from build123d import *

# Parameters (mm, degrees)
DODANIE_WYCI_GNI_CIE1_DEPTH   = 10
SZKIC1_W                      = 5
SZKIC1_H                      = 6
DODANIE_WYCI_GNI_CIE1_2_DEPTH = 10
DODANIE_WYCI_GNI_CIE1_3_DEPTH = 10
SZKIC1_3_W                    = 5
SZKIC1_3_H                    = 5
DODANIE_WYCI_GNI_CIE2_DEPTH   = 5
SZKIC2_R                      = 1
WYTNIJ_WYCI_GNI_CIE1_DEPTH    = 104.949507791


with BuildPart() as part:
    # Szkic1 → Dodanie-wyci_gni_cie1 (new body)
    with BuildSketch(Plane(origin=(0, 0, 0), x_dir=(1, 0, 0), z_dir=(0, 1, 0))):
        with BuildLine():
            Line((-9.449286184, 87.638462845), (9.449286184, 87.638462845))
            ThreePointArc((9.449286184, 87.638462845), (10.74338141, 87.468091977), (11.949286184, 86.968589864))
            Line((11.949286184, 86.968589864), (47.5, 66.443375673))
            ThreePointArc((47.5, 66.443375673), (49.330127019, 64.613248654), (50, 62.113248654))
            Line((50, 62.113248654), (50, 11))
            Line((50, 11), (55, 11))
            Line((55, 11), (55, 89.638462845))
            ThreePointArc((55, 89.638462845), (53.535533906, 93.173996751), (50, 94.638462845))
            Line((50, 94.638462845), (-50, 94.638462845))
            ThreePointArc((-50, 94.638462845), (-53.535533906, 93.173996751), (-55, 89.638462845))
            Line((-55, 89.638462845), (-55, 11))
            Line((-55, 11), (-50, 11))
            Line((-50, 11), (-50, 62.113248654))
            ThreePointArc((-50, 62.113248654), (-49.330127019, 64.613248654), (-47.5, 66.443375673))
            Line((-47.5, 66.443375673), (-11.949286184, 86.968589864))
            ThreePointArc((-11.949286184, 86.968589864), (-10.74338141, 87.468091977), (-9.449286184, 87.638462845))
        make_face()
        with BuildLine():
            ThreePointArc((-48.5, 70.620674679), (-49.5, 70.620674679), (-50, 71.486700083))
            Line((-50, 71.486700083), (-50, 86.638462845))
            ThreePointArc((-50, 86.638462845), (-49.707106781, 87.345569627), (-49, 87.638462845))
            Line((-49, 87.638462845), (-22.756377072, 87.638462845))
            ThreePointArc((-22.756377072, 87.638462845), (-21.790451246, 86.89728189), (-22.256377072, 85.772437442))
            Line((-22.256377072, 85.772437442), (-48.5, 70.620674679))
        make_face(mode=Mode.SUBTRACT)
        with BuildLine():
            Line((48.5, 70.620674679), (22.256377072, 85.772437442))
            ThreePointArc((22.256377072, 85.772437442), (21.790451246, 86.89728189), (22.756377072, 87.638462845))
            Line((22.756377072, 87.638462845), (49, 87.638462845))
            ThreePointArc((49, 87.638462845), (49.707106781, 87.345569627), (50, 86.638462845))
            Line((50, 86.638462845), (50, 71.486700083))
            ThreePointArc((50, 71.486700083), (49.5, 70.620674679), (48.5, 70.620674679))
        make_face(mode=Mode.SUBTRACT)
    extrude(amount=DODANIE_WYCI_GNI_CIE1_DEPTH)



with BuildPart() as body_2:
    # Szkic1 → Dodanie-wyci_gni_cie1 2 (new body)
    with BuildSketch(Plane(origin=(0, 0, 0), x_dir=(1, 0, 0), z_dir=(0, 1, 0))):
        with Locations((52.5, 3)):
            Rectangle(SZKIC1_W, SZKIC1_H)
    extrude(amount=DODANIE_WYCI_GNI_CIE1_2_DEPTH)


with BuildPart() as body_3:
    # Szkic1 → Dodanie-wyci_gni_cie1 3 (new body)
    with BuildSketch(Plane(origin=(0, 0, 0), x_dir=(1, 0, 0), z_dir=(0, 1, 0))):
        with Locations((-52.5, 3)):
            Rectangle(SZKIC1_W, SZKIC1_H)
    extrude(amount=DODANIE_WYCI_GNI_CIE1_3_DEPTH)


with BuildPart() as part_1:
    add(part.part)

    add(body_2.part)  # Dodanie-wyci_gni_cie2 merges body 2

    add(body_3.part)  # Dodanie-wyci_gni_cie2 merges body 3
    # Szkic1_3 → Dodanie-wyci_gni_cie2 (add)
    with BuildSketch(Plane(origin=(0, 0, 0), x_dir=(1, 0, 0), z_dir=(0, 1, 0))):
        with Locations((-52.5, 8.5)):
            Rectangle(SZKIC1_3_W, SZKIC1_3_H)
        with Locations((52.5, 8.5)):
            Rectangle(SZKIC1_3_W, SZKIC1_3_H)
    extrude(amount=DODANIE_WYCI_GNI_CIE2_DEPTH)

    # Szkic2 → Wytnij-wyci_gni_cie1 (cut, through all)
    with BuildSketch(Plane.XY.offset(-87.638462845)):
        with Locations((0, 5)):
            Circle(SZKIC2_R)
    extrude(amount=-WYTNIJ_WYCI_GNI_CIE1_DEPTH, mode=Mode.SUBTRACT)


solid = part_1.part
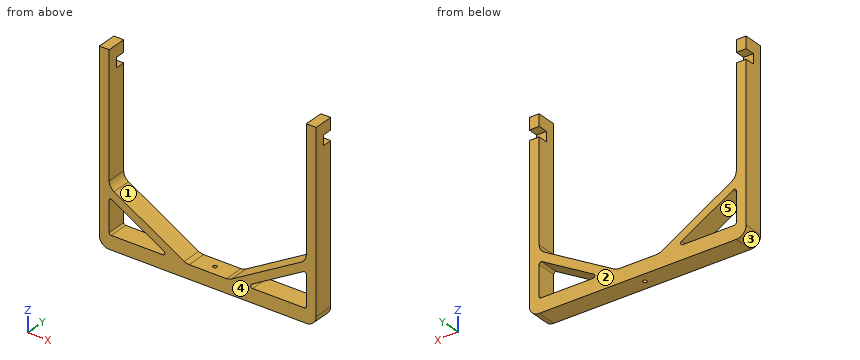
Work out the finished part from the listing and answer in its coordinate system (mm). Face numbers are marked on the shaded views. A direction names the side the tool comes from. Round coordinates to 2 decimals unless told otherwise and drop trailing zeros. Write each loop counter-clockwise with the first axis right and the second up, starting at its lowest first coordinate (ties: lowest second). Pieces come first, ordered by that corner, then holes. Notation, with made-up numbers: (21, 86.5) -> (69, 86.5) arc R19 cw to (69, 90.5) -> close; hole circle Ø11 at (-13, -26). An arc over 180 degrees is marked (long way). Answer as CSV lines item,"result". Start each with the question number.
(1) Each of these flat-tipped pins is pushed along its axis until it touches: pin 1 (1.5 mm diameter, centred on x = 52.5, y = 7, fed in from -Z); pin 2 (6 mm diameter, centred on x = -29.5, y = 4.5, fed in from +Z); pin 3 (5 mm diameter, centred on x = -1, y = 3.5, fed in from +Z). Where does it stop, or does it pass through?
(2) The part is cut by section C-C, the plane x = 4.5. Give the vertices of the cut face in (y, z), then the cut area to 3 significant figures.
(3) A tool of negligible diameter and unlimited length cuts with its end or side. For the marked faces 1 and 2, from which of +Z, -Z, +X, -X, +Y, -Y can it reach the whole face along a straight path? Write none if from no direction.
(4) The part is cut by section A-A, the plane z = -32. Give the vertices of the cut face in (x, y).
(5) The part is cut by section B-B, the plane z = -79. Give the vertices of the cut face in (x, y).
(6) The mould has two halves that part along X. Classify the marked faces 3, 4 and 5: +X half, -X half, draft (parallel to the pull), parting line (faces both ways), or undercut.
(7) Find the intervals of material crossed by probe 1 along X at (y, z) = (8.75, -43.5); probe 2 along Y at (x, z) = (0, -92); probe 3 along X at (y, z) = (9, -84), in increasing order.
(8) The part is cut by section D-D, the plane z = -63.5. Give the vertices of the cut face in (x, y), then the cut area to 3 significant figures.
Output values:
1,pin 1,"stops at z = -94.32"
1,pin 2,"stops at z = -75.1"
1,pin 3,"stops at z = -87.64"
2,outline,"(0, -94.64) -> (10, -94.64) -> (10, -87.64) -> (0, -87.64) -> close"
2,area,"70.0 mm²"
3,face 1,"+Z, +Y, -Y"
3,face 2,"+Z, -Z, +X, -X, +Y"
4,outline,"(-55, 0) -> (-50, 0) -> (-50, 10) -> (-55, 10) -> close; (50, 0) -> (55, 0) -> (55, 10) -> (50, 10) -> close"
5,outline,"(-55, 0) -> (-50, 0) -> (-50, 10) -> (-55, 10) -> close; (-33.99, 0) -> (-25.75, 0) -> (-25.75, 10) -> (-33.99, 10) -> close; (25.75, 0) -> (33.99, 0) -> (33.99, 10) -> (25.75, 10) -> close; (50, 0) -> (55, 0) -> (55, 10) -> (50, 10) -> close"
6,face 3,"-X half"
6,face 4,"draft"
6,face 5,"undercut"
7,probe 1,"x = -55 to -50, 50 to 55"
7,probe 2,"y = 0 to 4, 6 to 10"
7,probe 3,"x = -55 to -50, -25.33 to -17.09, 17.09 to 25.33, 50 to 55"
8,outline,"(-55, 0) -> (-49.8, 0) -> (-49.8, 10) -> (-55, 10) -> close; (49.8, 0) -> (55, 0) -> (55, 10) -> (49.8, 10) -> close"
8,area,"104 mm²"
